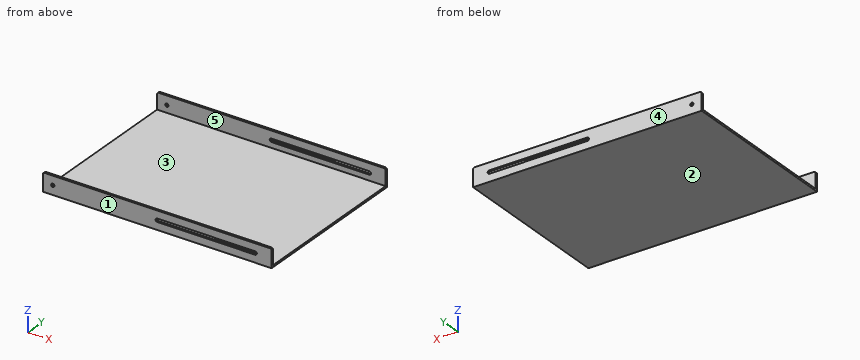
```python
from build123d import *

# Parameters (mm, degrees)
SKETCH4_R               = 5
BOSS_EXTRUDE2_DEPTH     = 256
CUT_EXTRUDE2_DEPTH      = 746.868621139
CUT_EXTRUDE2_DEPTH_BACK = 746.868621139
SKETCH5_W               = 50
SKETCH5_H               = 500


with BuildPart() as part:
    # Sketch4 → Boss-Extrude2 (new, symmetric)
    with BuildSketch(Plane(origin=(0, 0, 0), x_dir=(1, 0, 0), z_dir=(0, 1, 0))):
        with BuildLine():
            Line((-350, 28), (350, 28))
            Line((350, 28), (350, -23))
            ThreePointArc((350, -23), (348.535533906, -26.535533906), (345, -28))
            Line((345, -28), (-345, -28))
            ThreePointArc((-345, -28), (-348.535533906, -26.535533906), (-350, -23))
            Line((-350, -23), (-350, 28))
        make_face()
        with Locations(Location((-320, 0, 0), (0, 0, 270))):
            Circle(SKETCH4_R, mode=Mode.SUBTRACT)
        with BuildLine():
            Line((0, 5), (300, 5))
            ThreePointArc((300, 5), (305, 0), (300, -5))
            Line((300, -5), (0, -5))
            ThreePointArc((0, -5), (-5, 0), (0, 5))
        make_face(mode=Mode.SUBTRACT)
    extrude(amount=BOSS_EXTRUDE2_DEPTH, both=True)

    # Sketch5 → Cut-Extrude2 (cut, two sides: drawn at the far end of the back side and taken through both)
    with BuildSketch(Plane(origin=(350, 0, 0), x_dir=(0, 0, -1), z_dir=(1, 0, 0)).offset(-CUT_EXTRUDE2_DEPTH_BACK)):
        with Locations((-3, 0)):
            Rectangle(SKETCH5_W, SKETCH5_H)
    extrude(amount=CUT_EXTRUDE2_DEPTH + CUT_EXTRUDE2_DEPTH_BACK, mode=Mode.SUBTRACT)


solid = part.part
```
The model under review builds one solid part; all positions refer to its coordinate system, in mm. Face numbers are marked on the shaded views. A direction names the side the tool comes from. Round coordinates to 2 decimals unless told otherwise and drop trailing zeros. Order: outer loops, then holes, each group sorted by start corner. A loop starts at its lowest first (then second) coordinate and runs counter-clockwise, first axis right, second up. Notation, with made-up numbers: (-31, 78.5) -> (26, 78.5) arc R19 cw to (26, 86.5) -> close; hole circle Ø8 at (49, -11). An arc over 180 degrees is marked (long way). Use a Markdown table: item, result.
Q1. We need section C-C on y = -84.5. Write out the cut boundary in (x, z).
Values:
| item | result |
|---|---|
| outline | (-350, -28) -> (350, -28) -> (350, -22) -> (-350, -22) -> close |
Q2. Mouldability with a two-part tool opening along Y and no side actions: class the marked faces 1, 2 and 3 as +Y half, -Y half, draft (parallel to the pull), parting line (faces both ways), or undercut.
Values:
| item | result |
|---|---|
| face 1 | -Y half |
| face 2 | draft |
| face 3 | undercut |
Q3. Tool access review of the marked faces 4 and 5: name each direction out of +Z, -Z, +X, -X, +Y, -Y from which nothing blocks a thin tool from reaching the whole face with its end or side.
Values:
| item | result |
|---|---|
| face 4 | +Z, -Z, +X, -X, +Y |
| face 5 | +Z, +X, -X |
Q4. We need section B-B on x = -157.5. Write out the cut boundary in (y, z), then the cut area to 3 significant figures.
Values:
| item | result |
|---|---|
| outline | (-256, -28) -> (256, -28) -> (256, 28) -> (250, 28) -> (250, -22) -> (-250, -22) -> (-250, 28) -> (-256, 28) -> close |
| area | 3,670 mm^2 |
Q5. For line 1 (X direction, y = -253.45, z = 0); line 2 (Y direction, x = -79, z = -7.5); line 3 (Z direction, x = -320, y = 253.6), list the stretches that pass through material, from the lowest coordinate up.
Values:
| item | result |
|---|---|
| line 1 | x = -350 to -325, -315 to -5, 305 to 350 |
| line 2 | y = -256 to -250, 250 to 256 |
| line 3 | z = -28 to -5, 5 to 28 |
Q6. Clearance check with flat-ended pins moving along their axes: P1, Ø6, axis at x = -320, z = 0, coming from the -Y side; P2, Ø6, axis at x = 111.5, y = 78.5, coming from the +Z side; P3, Ø11.5, axis at x = -320, z = 0, coming from the +Y side. State where each tip first meets the part, or that it passes through.
Values:
| item | result |
|---|---|
| P1 | passes through |
| P2 | stops at z = -22 |
| P3 | stops at y = 256 |
Q7. We need section A-A on x = 61.5. Write out the cut boundary in (y, z), then the cut area to 3 significant figures.
Values:
| item | result |
|---|---|
| outline | (-256, -28) -> (256, -28) -> (256, -5) -> (250, -5) -> (250, -22) -> (-250, -22) -> (-250, -5) -> (-256, -5) -> close; (-256, 5) -> (-250, 5) -> (-250, 28) -> (-256, 28) -> close; (250, 5) -> (256, 5) -> (256, 28) -> (250, 28) -> close |
| area | 3,550 mm^2 |
